Can you work these out from the model? Positions are in its coordinate system, mm. Face numbers are marked on the shaded views. A direction names the side the tool comes from. Coordinates: 2 decimals unless noted, no trailing zeros. Loops run counter-clockwise (first coordinate to the right, second up) from the corner with the lowest first, then second, coordinate; pieces in that order, holes last. Notation, with made-up numbers: (52, -10.5) -> (71, -10.5) arc R17 cw to (71, 16.5) -> close; hole circle Ø2 at (78, -6.75). An arc over 180 degrees is marked (long way). Use one line per item in the form item = value. Start each with the question number.
(1) On a 3-axis mill with a long thin cutter (end or side, diameter ignored), from which of +Z, -Z, +X, -X, +Y, -Y can I reach the whole of each face in a straight line? I mean the marked faces 1 and 2. Say none if no direction works.
(2) Imagine slicing it at B-B (z = 92.5). List the corners of the cut face in (x, y) for me.
(3) I need wall thicknesses on line 1 (Z direction, x = 12, y = 1); line 2 (X direction, y = 1, z = 60); line 3 (Z direction, x = 102.5, y = 21). Which ranges of each line are inside material? Lowest first, please. Write a range as [from, to].
(4) Imagine slicing it at A-A (y = 12). List the corners of the cut face in (x, z) for me, plus the area to 3 significant figures.
(5) Thinking about a two-plate mould opening in Z: for the marked faces 3, 4, 5 and 6, which applies, released by +Z, released by -Z, zero draft, split by the parting line, or undercut?
(6) Imagine slicing it at C-C (x = 39.7). List the corners of the cut face in (y, z) for me, plus the area to 3 significant figures.
(7) Imagine slicing it at D-D (x = 12.7). List the corners of the cut face in (y, z) for me, plus the area to 3 significant figures.
(8) I'm going to push a flat-ended pin straight in: pin 1 (13.5 mm diameter, centred on x = 12.7, z = 60.3, fed in from +Y). Where does the tip first touch, or does it pass through?
```python
from build123d import *

# Parameters (mm, degrees)
SKETCH1_W           = 139.7
SKETCH1_H           = 111.1
SKETCH1_R           = 5.15
BOSS_EXTRUDE1_DEPTH = 4.8
SKETCH1_4_W         = 139.7
SKETCH1_4_H         = 4.8
BOSS_EXTRUDE2_DEPTH = 149


with BuildPart() as part:
    # Sketch1 → Boss-Extrude1 (new body)
    with BuildSketch(Plane(origin=(0, 0, 0), x_dir=(1, 0, 0), z_dir=(0, 1, 0))):
        with Locations((69.85, -60.35)):
            Rectangle(SKETCH1_W, SKETCH1_H)
        with BuildLine():
            ThreePointArc((7.55, -87.3), (12.7, -82.15), (17.85, -87.3))
            Line((17.85, -87.3), (17.85, -100))
            ThreePointArc((17.85, -100), (12.7, -105.15), (7.55, -100))
            Line((7.55, -100), (7.55, -87.3))
        make_face(mode=Mode.SUBTRACT)
        with Locations(Location((12.7, -60.3, 0), (0, 0, 270))):
            Circle(SKETCH1_R, mode=Mode.SUBTRACT)
        with Locations(Location((39.7, -60.3, 0), (0, 0, 270))):
            Circle(SKETCH1_R, mode=Mode.SUBTRACT)
        with BuildLine():
            Line((7.55, -33.3), (7.55, -20.6))
            ThreePointArc((7.55, -20.6), (12.7, -15.45), (17.85, -20.6))
            Line((17.85, -20.6), (17.85, -33.3))
            ThreePointArc((17.85, -33.3), (12.7, -38.45), (7.55, -33.3))
        make_face(mode=Mode.SUBTRACT)
        with BuildLine():
            ThreePointArc((92.1, -65.45), (86.95, -60.3), (92.1, -55.15))
            Line((92.1, -55.15), (123.9, -55.15))
            ThreePointArc((123.9, -55.15), (127.541599923, -56.658400077), (129.05, -60.3))
            ThreePointArc((129.05, -60.3), (127.541599923, -63.941599923), (123.9, -65.45))
            Line((123.9, -65.45), (92.1, -65.45))
        make_face(mode=Mode.SUBTRACT)
    extrude(amount=BOSS_EXTRUDE1_DEPTH)

    # Sketch1_4 → Boss-Extrude2 (add)
    with BuildSketch(Plane(origin=(0, 0, 0), x_dir=(1, 0, 0), z_dir=(0, 1, 0))):
        with Locations((69.85, -118.3)):
            Rectangle(SKETCH1_4_W, SKETCH1_4_H)
        with Locations((69.85, -2.4)):
            Rectangle(SKETCH1_4_W, SKETCH1_4_H)
    extrude(amount=BOSS_EXTRUDE2_DEPTH)


solid = part.part
```
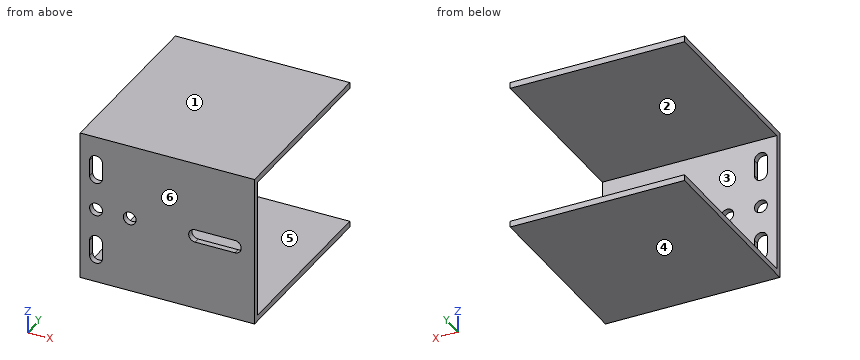
Worked out:
q1.face_1 = +Z, +X, -X, +Y, -Y
q1.face_2 = +X, -X, +Y
q2.outline = (0, 0) -> (7.55, 0) -> (7.55, 4.8) -> (0, 4.8) -> close; (17.85, 0) -> (139.7, 0) -> (139.7, 4.8) -> (17.85, 4.8) -> close
q3.line_1 = [0, 15.5], [38.4, 55.2], [65.4, 82.2], [105.1, 120.7]
q3.line_2 = [0, 7.56], [17.84, 34.56], [44.84, 86.96], [129.04, 139.7]
q3.line_3 = [0, 4.8], [115.9, 120.7]
q4.outline = (0, 0) -> (139.7, 0) -> (139.7, 4.8) -> (0, 4.8) -> close; (0, 115.9) -> (139.7, 115.9) -> (139.7, 120.7) -> (0, 120.7) -> close
q4.area = 1,340 mm2
q5.face_3 = undercut
q5.face_4 = released by -Z
q5.face_5 = undercut
q5.face_6 = zero draft
q6.outline = (0, 0) -> (149, 0) -> (149, 4.8) -> (4.8, 4.8) -> (4.8, 55.15) -> (0, 55.15) -> close; (0, 65.45) -> (4.8, 65.45) -> (4.8, 115.9) -> (149, 115.9) -> (149, 120.7) -> (0, 120.7) -> close
q6.area = 1,910 mm2
q7.outline = (0, 0) -> (149, 0) -> (149, 4.8) -> (4.8, 4.8) -> (4.8, 15.45) -> (0, 15.45) -> close; (0, 38.45) -> (4.8, 38.45) -> (4.8, 55.15) -> (0, 55.15) -> close; (0, 65.45) -> (4.8, 65.45) -> (4.8, 82.15) -> (0, 82.15) -> close; (0, 105.15) -> (4.8, 105.15) -> (4.8, 115.9) -> (149, 115.9) -> (149, 120.7) -> (0, 120.7) -> close
q7.area = 1,690 mm2
q8.pin_1 = 4.8
